from build123d import *

# Parameters (mm, degrees)
ESBO_O1_W                = 70
ESBO_O1_H                = 8
ESBO_O1_R                = 1.75
RESSALTO_EXTRUS_O1_DEPTH = 4
RESSALTO_EXTRUS_O2_DEPTH = 8


with BuildPart() as part:
    # Esboço1 → Ressalto-extrusão1 (new body)
    with BuildSketch(Plane.XY):
        Rectangle(ESBO_O1_W, ESBO_O1_H)
        with Locations((-31, 0)):
            Circle(ESBO_O1_R, mode=Mode.SUBTRACT)
        with Locations((31, 0)):
            Circle(ESBO_O1_R, mode=Mode.SUBTRACT)
    extrude(amount=RESSALTO_EXTRUS_O1_DEPTH)

    # Esboço2 → Ressalto-extrusão2 (add)
    with BuildSketch(Plane(origin=(0, 4, 0), x_dir=(1, 0, 0), z_dir=(0, 1, 0))):
        Polygon((-35, 0), (-35, -4), (-39.018745266, -4), (-39.018745266, 0), (-34.25, 49.2), (-28.25, 49.2), (-28.25, 47.2), (-30.25, 47.2), (-30.25, 45), (-28.25, 45), (-28.25, 43), (-30.832194178, 43), align=None)
        Polygon((39.018745266, -4), (35, -4), (35, 0), (30.832194178, 43), (28.25, 43), (28.25, 45), (30.25, 45), (30.25, 47.2), (28.25, 47.2), (28.25, 49.2), (34.25, 49.2), (39.018745266, 0), align=None)
    extrude(amount=-RESSALTO_EXTRUS_O2_DEPTH)


solid = part.part
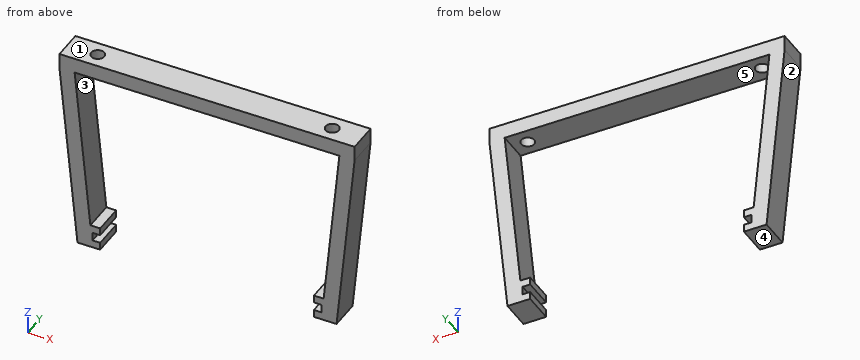
The listing builds one solid part. Answer for the finished solid, in the listing's coordinates (mm). Face numbers are marked on the shaded views. A direction names the side the tool comes from. Coordinates: 2 decimals unless noted, no trailing zeros. Write each loop counter-clockwise with the first axis right and the second up, starting at its lowest first coordinate (ties: lowest second). Pieces come first, ordered by that corner, then holes. Notation, with made-up numbers: (32.25, 71) - (45.25, 71) arc R8 ccw to (45.25, 86) - close; hole circle Ø9 at (-14.5, 67.5). An arc over 180 degrees is marked (long way). Answer as CSV lines item,"result".
1. Given P1, Ø1.6, axis at y = 0.5, z = -48, coming from the +X side; P2, Ø1.1, axis at y = -1.5, z = -46.5, coming from the -X side (3 decimals); P3, Ø0.7, axis at y = 0, z = -46, coming from the +X side; P4, Ø6, axis at x = 28, z = -33.5, coming from the +Y side, each flat-ended and moving along its own axis, determine where each tip first touches the part or whether it passes through.
Computed values:
P1,"stops at x = 34.44"
P2,"stops at x = -34.565"
P3,"stops at x = 34.59"
P4,"passes through"
2. A tool of negligible diameter and unlimited length cuts with its end or side. For the marked faces 4 and 5, from which of +Z, -Z, +X, -X, +Y, -Y can it reach the whole face along a straight path? Write none if from no direction.
Computed values:
face 4,"-Z, +X, -X, +Y, -Y"
face 5,"+Y, -Y"
3. Find section C-C (x = 23). Give the vertices of the cut face in (y, z).
Computed values:
outline,"(-4, 0) - (4, 0) - (4, 4) - (-4, 4) - close"
4. Straight lines are drawn through the part: line 1 (Z direction, x = -29.5, y = 3.25); line 2 (Y direction, x = 31, z = 2.55); line 3 (Z direction, x = 22, y = -3). For each, find the intervals that lie inside material, in ascending order. Write a range as [from, to].
Computed values:
line 1,"z = [-49.2, -47.2], [-45, -43], [0, 4]"
line 2,"y = [-4, -1.75], [1.75, 4]"
line 3,"z = [0, 4]"
5. Find section B-B (z = -10.5). Give the vertices of the cut face in (x, y), plus the area to 3 significant figures.
Computed values:
outline,"(-38, -4) - (-33.98, -4) - (-33.98, 4) - (-38, 4) - close; (33.98, -4) - (38, -4) - (38, 4) - (33.98, 4) - close"
area,"64.3 mm²"
6. Determine the mould class of the marked faces 1, 2 and 3 for opening direction X: +X half, -X half, draft (parallel to the pull), parting line (faces both ways), or undercut.
Computed values:
face 1,"draft"
face 2,"-X half"
face 3,"undercut"
7. Find section A-A (y = 0). Give the number of separate pieces and of enclosed holes in the cut face, plus the area to 3 significant figures.
Computed values:
separate pieces,"3"
enclosed holes,"0"
area,"699 mm²"
